Can you work these out from the model? Positions are in its coordinate system, mm. A direction names the side the tool comes from. Give positions to 0.01 mm unless a question says otherwise; leave off trailing zeros. Write each loop counter-clockwise with the first axis right and the second up, starting at its lowest first coordinate (ties: lowest second). Pieces come first, ordered by that corner, then holes. Notation, with made-up numbers: (-27.75, 73.25) -> (31.25, 73.25) arc R23 ccw to (31.25, 111.25) -> close; hole circle Ø11 at (-9.5, 51.5). An arc over 180 degrees is marked (long way). Answer as CSV lines item,"result". Start each with the question number.
1. If we mould it in two halves opening along Z, with no side actions, what happens to faces 3 (the face through (-84.945, -0.021, -94.429)), 4 (the face through (84.945, 0.021, 94.429)), 5 (the face through (-1, -1.5, -1))? For each: pulls with the +Z half, pulls with the -Z half, needs draft (parallel to the pull), parting line crosses it, or undercut.
2. If we section it at A-A on z = -36: Write out the boundary of the cut face in (x, y).
3. I'm going to push a flat-ended pin straight in: P1, Ø2.5, axis at x = -24.5, z = 17.5, coming from the +Y side. Where does the tip first touch, or does it pass through?
4. I need wall thicknesses on line 1 (Z direction, x = 24.5, y = -0.6); line 2 (Z direction, x = 3, y = 0.4); line 3 (X direction, y = 0.65, z = -37.5). Which ranges of each line are inside material? Lowest first, please. Write a range as [from, to].
5. If we section it at C-C on y = 0: Count the separate pieces of the cut face and the enclosed holes in it, plus the area to 3 significant figures.
6. If we section it at B-B on x = 18.5: Write out the boundary of the cut face in (y, z), plus the area to 3 significant figures.
7. On a 3-axis mill with a long thin cutter (end or side, diameter ignored), from which of +Z, -Z, +X, -X, +Y, -Y can I reach the whole of each face in a straight line? I mean faces 1 (the face through (16.85, -0.02, -100.44)), 2 (the face through (84.945, -0.021, -94.429)). Say none if no direction works.
```python
from build123d import *

# Parameters (mm, degrees)
SKETCH1_W                = 187
SKETCH1_H                = 206.9
BOSS_EXTRUDE1_DEPTH      = 1.5
FILLET1_R                = 30
SKETCH2_W                = 3
SKETCH2_H                = 30
CUT_EXTRUDE1_DEPTH       = 2.5
CUT_EXTRUDE1_DEPTH_BACK  = 2.5
SKETCH4_R                = 1.35
CUT_EXTRUDE3_DEPTH       = 1
CUT_EXTRUDE3_DEPTH_BACK  = 4
CUT_EXTRUDE2_DEPTH       = 4
CUT_EXTRUDE5_DEPTH       = 1
CUT_EXTRUDE5_DEPTH_BACK  = 4
CUT_EXTRUDE6_DEPTH       = 2.5
CUT_EXTRUDE6_DEPTH_BACK  = 2.5
SKETCH10_R               = 1.5
CUT_EXTRUDE9_DEPTH       = 2.5
CUT_EXTRUDE9_DEPTH_BACK  = 2.5
SKETCH11_W               = 28
SKETCH11_H               = 30.45294386
CUT_EXTRUDE10_DEPTH      = 1
CUT_EXTRUDE10_DEPTH_BACK = 4
FILLET2_R                = 10
FILLET2_2_R              = 1
SKETCH12_W               = 12
SKETCH12_H               = 3
CUT_EXTRUDE11_DEPTH      = 2.5
CUT_EXTRUDE11_DEPTH_BACK = 2.5


with BuildPart() as part:
    # Sketch1 → Boss-Extrude1 (new body, symmetric)
    with BuildSketch(Plane(origin=(0, 0, 0), x_dir=(1, 0, 0), z_dir=(0, 1, 0))):
        Rectangle(SKETCH1_W, SKETCH1_H)
    extrude(amount=BOSS_EXTRUDE1_DEPTH, both=True)

    # Fillet1
    fillet1_edges = [part.edges().sort_by_distance(p)[0] for p in [
        (-93.5, 0, -103.45),
        (93.5, 0, -103.45),
        (93.5, 0, 103.45),
        (-93.5, 0, 103.45),
    ]]
    fillet(fillet1_edges, radius=FILLET1_R)

    # Sketch2 → Cut-Extrude1 (cut, two sides)
    with BuildSketch(Plane(origin=(0, 0, 0), x_dir=(1, 0, 0), z_dir=(0, 1, 0))) as cut_extrude1_sk:
        with Locations((-51.5, 35)):
            Rectangle(SKETCH2_W, SKETCH2_H)
        with Locations((-51.5, -35)):
            Rectangle(SKETCH2_W, SKETCH2_H)
        with Locations((51.5, -35)):
            Rectangle(SKETCH2_W, SKETCH2_H)
        with Locations((51.5, 35)):
            Rectangle(SKETCH2_W, SKETCH2_H)
    extrude(amount=CUT_EXTRUDE1_DEPTH, mode=Mode.SUBTRACT)
    extrude(cut_extrude1_sk.sketch, amount=-CUT_EXTRUDE1_DEPTH_BACK, mode=Mode.SUBTRACT)

    # Sketch4 → Cut-Extrude3 (cut, two sides)
    with BuildSketch(Plane(origin=(0, 1.5, 0), x_dir=(1, 0, 0), z_dir=(0, 1, 0))) as cut_extrude3_sk:
        with Locations((24.5, -17.5)):
            Circle(SKETCH4_R)
        with Locations((-24.5, -17.5)):
            Circle(SKETCH4_R)
        with Locations((24.5, 40.5)):
            Circle(SKETCH4_R)
        with Locations((-24.5, 40.5)):
            Circle(SKETCH4_R)
    extrude(amount=CUT_EXTRUDE3_DEPTH, mode=Mode.SUBTRACT)
    extrude(cut_extrude3_sk.sketch, amount=-CUT_EXTRUDE3_DEPTH_BACK, mode=Mode.SUBTRACT)

    # Sketch3 → Cut-Extrude2 (cut, through all)
    with BuildSketch(Plane(origin=(0, 1.5, 0), x_dir=(1, 0, 0), z_dir=(0, 1, 0))):
        with BuildLine():
            Line((50, 45.75), (50, 24.25))
            Line((50, 24.25), (35.5, 24.25))
            ThreePointArc((35.5, 24.25), (34.085786438, 24.835786438), (33.5, 26.25))
            Line((33.5, 26.25), (33.5, 43.75))
            ThreePointArc((33.5, 43.75), (34.085786438, 45.164213562), (35.5, 45.75))
            Line((35.5, 45.75), (50, 45.75))
        make_face()
    extrude(amount=-CUT_EXTRUDE2_DEPTH, mode=Mode.SUBTRACT)

    # Sketch6 → Cut-Extrude5 (cut, two sides)
    with BuildSketch(Plane(origin=(0, 1.5, 0), x_dir=(1, 0, 0), z_dir=(0, 1, 0))) as cut_extrude5_sk:
        with BuildLine():
            Line((-25.2, -47.73), (25.2, -47.73))
            ThreePointArc((25.2, -47.73), (25.907106781, -48.022893219), (26.2, -48.73))
            Line((26.2, -48.73), (26.2, -62.73))
            ThreePointArc((26.2, -62.73), (25.907106781, -63.437106781), (25.2, -63.73))
            Line((25.2, -63.73), (-25.2, -63.73))
            ThreePointArc((-25.2, -63.73), (-25.907106781, -63.437106781), (-26.2, -62.73))
            Line((-26.2, -62.73), (-26.2, -48.73))
            ThreePointArc((-26.2, -48.73), (-25.907106781, -48.022893219), (-25.2, -47.73))
        make_face()
    extrude(amount=CUT_EXTRUDE5_DEPTH, mode=Mode.SUBTRACT)
    extrude(cut_extrude5_sk.sketch, amount=-CUT_EXTRUDE5_DEPTH_BACK, mode=Mode.SUBTRACT)

    # Sketch7 → Cut-Extrude6 (cut, two sides)
    with BuildSketch(Plane(origin=(0, 0, 0), x_dir=(1, 0, 0), z_dir=(0, 1, 0))) as cut_extrude6_sk:
        with BuildLine():
            Line((-24.85, 52.23), (24.85, 52.23))
            ThreePointArc((24.85, 52.23), (25.557106781, 51.937106781), (25.85, 51.23))
            Line((25.85, 51.23), (25.85, 45.85))
            ThreePointArc((25.85, 45.85), (25.557106781, 45.142893219), (24.85, 44.85))
            Line((24.85, 44.85), (-24.85, 44.85))
            ThreePointArc((-24.85, 44.85), (-25.557106781, 45.142893219), (-25.85, 45.85))
            Line((-25.85, 45.85), (-25.85, 51.23))
            ThreePointArc((-25.85, 51.23), (-25.557106781, 51.937106781), (-24.85, 52.23))
        make_face()
    extrude(amount=CUT_EXTRUDE6_DEPTH, mode=Mode.SUBTRACT)
    extrude(cut_extrude6_sk.sketch, amount=-CUT_EXTRUDE6_DEPTH_BACK, mode=Mode.SUBTRACT)

    # Sketch10 → Cut-Extrude9 (cut, two sides)
    with BuildSketch(Plane(origin=(0, 0, 0), x_dir=(1, 0, 0), z_dir=(0, 1, 0))) as cut_extrude9_sk:
        with Locations((-80.35, 0)):
            Circle(SKETCH10_R)
        with Locations((80.35, 0)):
            Circle(SKETCH10_R)
    extrude(amount=CUT_EXTRUDE9_DEPTH, mode=Mode.SUBTRACT)
    extrude(cut_extrude9_sk.sketch, amount=-CUT_EXTRUDE9_DEPTH_BACK, mode=Mode.SUBTRACT)

    # Sketch11 → Cut-Extrude10 (cut, two sides)
    with BuildSketch(Plane(origin=(0, 1.5, 0), x_dir=(1, 0, 0), z_dir=(0, 1, 0))) as cut_extrude10_sk:
        with Locations((0, 88.22352807)):
            Rectangle(SKETCH11_W, SKETCH11_H)
    extrude(amount=CUT_EXTRUDE10_DEPTH, mode=Mode.SUBTRACT)
    extrude(cut_extrude10_sk.sketch, amount=-CUT_EXTRUDE10_DEPTH_BACK, mode=Mode.SUBTRACT)

    # Fillet2
    fillet2_edges = [part.edges().sort_by_distance(p)[0] for p in [
        (-14, 0, -103.45),
        (14, 0, -103.45),
    ]]
    fillet(fillet2_edges, radius=FILLET2_R)

    # Fillet2 2
    fillet2_2_edges = [part.edges().sort_by_distance(p)[0] for p in [
        (-14, 0, -72.99705614),
        (14, 0, -72.99705614),
    ]]
    fillet(fillet2_2_edges, radius=FILLET2_2_R)

    # Sketch12 → Cut-Extrude11 (cut, two sides)
    with BuildSketch(Plane(origin=(0, 0, 0), x_dir=(1, 0, 0), z_dir=(0, 1, 0))) as cut_extrude11_sk:
        with Locations((0, 71.49705614)):
            Rectangle(SKETCH12_W, SKETCH12_H)
    extrude(amount=CUT_EXTRUDE11_DEPTH, mode=Mode.SUBTRACT)
    extrude(cut_extrude11_sk.sketch, amount=-CUT_EXTRUDE11_DEPTH_BACK, mode=Mode.SUBTRACT)


solid = part.part
```
Computed values:
1,face 3,"pulls with the -Z half"
1,face 4,"pulls with the +Z half"
1,face 5,"needs draft"
2,outline,"(-93.5, -1.5) -> (-53, -1.5) -> (-53, 1.5) -> (-93.5, 1.5) -> close; (-50, -1.5) -> (33.5, -1.5) -> (33.5, 1.5) -> (-50, 1.5) -> close; (53, -1.5) -> (93.5, -1.5) -> (93.5, 1.5) -> (53, 1.5) -> close"
3,P1,"passes through"
4,line 1,"z = [-103.45, -52.23], [-44.85, -41.85], [-39.15, 16.15], [18.85, 47.73], [63.73, 103.45]"
4,line 2,"z = [-70, -52.23], [-44.85, 47.73], [63.73, 103.45]"
4,line 3,"x = [-93.5, -53], [-50, 33.5], [53, 93.5]"
5,separate pieces,"1"
5,enclosed holes,"12"
5,area,"35,000 mm2"
6,outline,"(-1.5, -101.8) -> (1.5, -101.8) -> (1.5, -52.23) -> (-1.5, -52.23) -> close; (-1.5, -44.85) -> (1.5, -44.85) -> (1.5, 47.73) -> (-1.5, 47.73) -> close; (-1.5, 63.73) -> (1.5, 63.73) -> (1.5, 103.45) -> (-1.5, 103.45) -> close"
6,area,"546 mm2"
7,face 1,"-Z, +Y, -Y"
7,face 2,"-Z, +X, +Y, -Y"
